Part print with two shaded views. Sizes in mm from the minimum x, y, z corner. Coordinates: 2 decimals unless noted, no trailing zeros. Answer in a Markdown table with one row per item. Add a question column.
Q1. Pin check, flat tip, straight feed: pin 1 (3 mm diameter, centred on x = 80, y = 60, fed in from -Z). Stop position of the tip, or through.
Q2. Band-saw the part on A-A (x = 50). State how many separate pieces and enclosed holes the cut face has, and give its area (3 significant figures).
Q3. Drill centre line: line 1 along Y through (x, z) = (4, 2.05). Where is it in solid material? Low to high. Write a range as from..to.
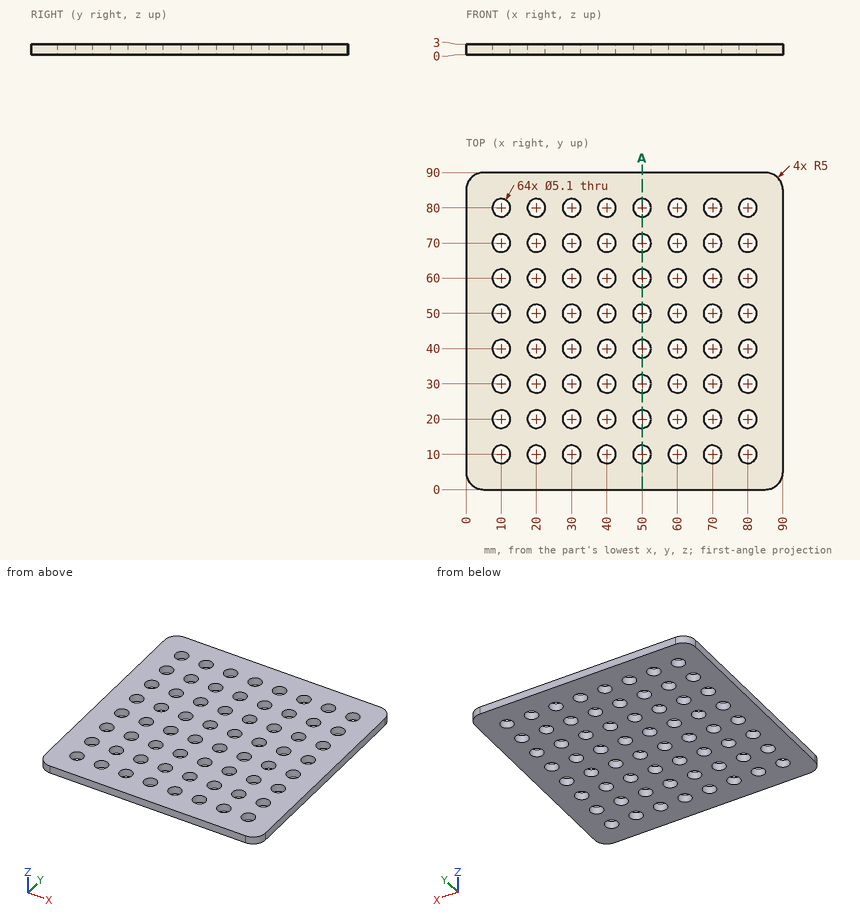
Checked values:
| question | item | result |
|---|---|---|
| 1 | pin 1 | passes through |
| 2 | separate pieces | 9 |
| 2 | enclosed holes | 0 |
| 2 | area | 148 mm² |
| 3 | line 1 | y = 0.1..89.9 |
